```python
from build123d import *

# Parameters (mm, degrees)
F1_DEPTH  = 9.652
F2_R      = 2.413
F3_DEPTH  = 1.778
F4_DEPTH  = 1.778
F5_DEPTH  = 1.778
F6_DEPTH  = 1.778
F7_T      = -1.778
F8_R      = 1.4417359586
F9_DEPTH  = 7.87157
F8_R_2    = 1.507368722
F10_DEPTH = 7.88241
F8_R_3    = 1.5366007798
F11_DEPTH = 7.85389


with BuildPart() as f1:
    # F0 (on Top) → F1 (new body)
    with BuildSketch(Plane.XY):
        Polygon((-7.874, 0), (0, 0), (23.622, 0), (23.622, 7.874), (-7.874, 7.874), align=None)
    extrude(amount=F1_DEPTH)

    # F2 (on face) → F3 (join)
    with BuildSketch(Plane.XY.offset(9.652)):
        with Locations((19.685, 3.937)):
            Circle(F2_R)
    extrude(amount=F3_DEPTH)

    # F2 (on face) → F4 (join)
    with BuildSketch(Plane.XY.offset(9.652)):
        with Locations((11.811, 3.937)):
            Circle(F2_R)
    extrude(amount=F4_DEPTH)

    # F2 (on face) → F5 (join)
    with BuildSketch(Plane.XY.offset(9.652)):
        with Locations((3.937, 3.937)):
            Circle(F2_R)
    extrude(amount=F5_DEPTH)

    # F2 (on face) → F6 (join)
    with BuildSketch(Plane.XY.offset(9.652)):
        with Locations((-3.937, 3.937)):
            Circle(F2_R)
    extrude(amount=F6_DEPTH)

    # F7
    f7_openings = [f1.faces().sort_by_distance(p)[0] for p in [
        (7.874, 3.937, 0),
    ]]
    offset(amount=F7_T, openings=f7_openings, kind=Kind.INTERSECTION)

    # F8 (on face) → F9 (join)
    with BuildSketch(Plane(origin=(0, 0, 7.874), x_dir=(1, 0, 0), z_dir=(0, 0, -1))):
        with Locations((15.8983748406, -4.0523083881)):
            Circle(F8_R)
    extrude(amount=F9_DEPTH)

    # F8 (on face) → F10 (join)
    with BuildSketch(Plane(origin=(0, 0, 7.874), x_dir=(1, 0, 0), z_dir=(0, 0, -1))):
        with Locations((8.1644477323, -4.0523083881)):
            Circle(F8_R_2)
    extrude(amount=F10_DEPTH)

    # F8 (on face) → F11 (join)
    with BuildSketch(Plane(origin=(0, 0, 7.874), x_dir=(1, 0, 0), z_dir=(0, 0, -1))):
        with Locations((0, -4.0523083881)):
            Circle(F8_R_3)
    extrude(amount=F11_DEPTH)


solid = f1.part
```
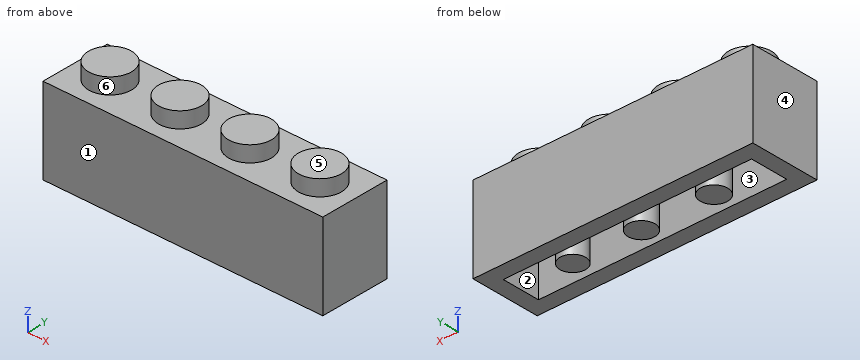
Geometry: final body of the model. Coordinates: model frame, mm. Face numbers are marked on the shaded views. A direction names the side the tool comes from. Round coordinates to 2 decimals unless told otherwise and drop trailing zeros. Write each loop counter-clockwise with the first axis right and the second up, starting at its lowest first coordinate (ties: lowest second). Pieces come first, ordered by that corner, then holes.
Item 1: Set-up query: the marked faces 5 and 6. Return all of +Z, -Z, +X, -X, +Y, -Y with unobstructed straight access to the full face (end or side cutting, diameter ignored); none if empty.
Item 2: Material intervals for L1, parallel to Y at x = 16, z = 1.5; L2, parallel to X at y = 1.75, z = 11.25; L3, parallel to X at y = 3.75, z = 3, sorted ascending.
Item 3: Section query A-A (z = 2). Return loops of the section in (x, y).
Item 4: Pin query (flat end, axial travel): P1, Ø0.8, axis at x = 19.685, y = 3.937, coming from the -Z side; P2, Ø1, axis at x = 20, y = 4, coming from the -Z side; P3, Ø0.9, axis at x = 16.5, y = 4, coming from the -Z side. Return the tip coordinate at first contact, or that it passes through.
Item 5: Mould query, pull axis Y, two halves, no side actions, for the marked faces 1, 2, 3 and 4. Classes: +Y half, -Y half, draft (parallel to the pull), parting line (faces both ways), or undercut.
Item 6: Section query B-B (x = 0). Return loops of the section in (y, z).
Item 7: Section query C-C (y = 6.75). Return loops of the section in (x, z), plus the area to 3 significant figures.
Item 8: Section query D-D (x = 18). Return loops of the section in (y, z).
Completed:
1. face 5: +Z, +X, -X, +Y, -Y
1. face 6: +Z
2. L1: y = 0 to 1.78, 2.61 to 5.49, 6.1 to 7.87
2. L2: x = -4.96 to -2.92, 2.92 to 4.96, 10.79 to 12.83, 18.67 to 20.7
2. L3: x = -7.87 to -6.1, -1.51 to 1.51, 6.69 to 9.64, 14.49 to 17.31, 21.84 to 23.62
3. outline: (-7.87, 0) - (23.62, 0) - (23.62, 7.87) - (-7.87, 7.87) - close; circle Ø3.07 at (0, 4.05); circle Ø3.01 at (8.16, 4.05); circle Ø2.88 at (15.9, 4.05); hole (-6.1, 1.78) - (21.84, 1.78) - (21.84, 6.1) - (-6.1, 6.1) - close
4. P1: stops at z = 9.65
4. P2: stops at z = 7.87
4. P3: stops at z = 0
5. face 1: -Y half
5. face 2: undercut
5. face 3: undercut
5. face 4: draft
6. outline: (0, 0) - (1.78, 0) - (1.78, 7.87) - (2.52, 7.87) - (2.52, 0.02) - (5.59, 0.02) - (5.59, 7.87) - (6.1, 7.87) - (6.1, 0) - (7.87, 0) - (7.87, 9.65) - (0, 9.65) - close
7. outline: (-7.87, 0) - (23.62, 0) - (23.62, 9.65) - (-7.87, 9.65) - close
7. area: 304 mm2
8. outline: (0, 0) - (1.78, 0) - (1.78, 7.87) - (6.1, 7.87) - (6.1, 0) - (7.87, 0) - (7.87, 9.65) - (5.66, 9.65) - (5.66, 11.43) - (2.21, 11.43) - (2.21, 9.65) - (0, 9.65) - close
